```python
from build123d import *

# Parameters (mm, degrees)
SKETCH1_W           = 20
SKETCH1_H           = 200
SKETCH1_R           = 2
BOSS_EXTRUDE1_DEPTH = 10.5


with BuildPart() as part:
    # Sketch1 → Boss-Extrude1 (new body)
    with BuildSketch(Plane(origin=(0, 0, 0), x_dir=(1, 0, 0), z_dir=(0, 1, 0))):
        Rectangle(SKETCH1_W, SKETCH1_H)
        with Locations((0, 80)):
            Circle(SKETCH1_R, mode=Mode.SUBTRACT)
        Circle(SKETCH1_R, mode=Mode.SUBTRACT)
        with Locations((0, -80)):
            Circle(SKETCH1_R, mode=Mode.SUBTRACT)
    extrude(amount=BOSS_EXTRUDE1_DEPTH)


solid = part.part
```
Geometry: final body of the model. Coordinates: model frame, mm. Coordinates: 2 decimals unless noted, no trailing zeros. Order: outer loops, then holes, each group sorted by start corner. A loop starts at its lowest first (then second) coordinate and runs counter-clockwise, first axis right, second up. Notation, with made-up numbers: M 35.5,-3 L 84.5,-3 A23 cw 84.5,17 Z; hole C 4,52 d8. An arc over 180 degrees is marked long. Answer as CSV lines item,"result".
Q1. Section A-A on x = 0. Return the cut outline in (y, z), and give its area (3 significant figures).
Answers:
outline,"M 0,-100 L 10.5,-100 L 10.5,-82 L 0,-82 Z; M 0,-78 L 10.5,-78 L 10.5,-2 L 0,-2 Z; M 0,2 L 10.5,2 L 10.5,78 L 0,78 Z; M 0,82 L 10.5,82 L 10.5,100 L 0,100 Z"
area,"1,970 mm^2"
Q2. Line query: probe 1 along Z at (x, y) = (0, 6.75); probe 2 along X at (y, z) = (8, 0); probe 3 along Z at (x, y) = (-1.5, 10). Output: solid intervals per line, ascending. Write a range as [from, to].
Answers:
probe 1,"z = [-100, -82], [-78, -2], [2, 78], [82, 100]"
probe 2,"x = [-10, -2], [2, 10]"
probe 3,"z = [-100, -81.32], [-78.68, -1.32], [1.32, 78.68], [81.32, 100]"
Q3. Section B-B on z = -80. Return the cut outline in (x, y).
Answers:
outline,"M -10,0 L -2,0 L -2,10.5 L -10,10.5 Z; M 2,0 L 10,0 L 10,10.5 L 2,10.5 Z"
Q4. Draft query along X for faces 1 (the flat face through (10, 5, 1)), 2 (the flat face through (0, 5, 100)), 3 (the cylindrical face through (0, 5, 78)). Return one class per face: pulls with the +X half, pulls with the -X half, needs draft (parallel to the pull), parting line crosses it, or undercut.
Answers:
face 1,"pulls with the +X half"
face 2,"needs draft"
face 3,"undercut"
Q5. First-contact query: P1, Ø3.5, axis at x = 0, z = 80, coming from the +Y side. Flat tip, straight axial feed; report the tip coordinate or a pass-through.
Answers:
P1,"passes through"
